```python
from build123d import *

# Parameters (mm, degrees)
SKETCH1_W            = 100
SKETCH1_H            = 100
BOSS_EXTRUDE1_DEPTH  = 5
SKETCH2_W            = 90
SKETCH2_H            = 90
SKETCH2_W_2          = 84
SKETCH2_H_2          = 84
BOSS_EXTRUDE2_DEPTH  = 10
SKETCH4_W            = 5
SKETCH4_H            = 5
SKETCH4_R            = 1.5
BOSS_EXTRUDE3_DEPTH  = 2
FILLET1_R            = 1
SKETCH5_W            = 60
SKETCH5_H            = 10
CUT_EXTRUDE1_DEPTH   = 5
SKETCH6_R            = 1.5
CUT_EXTRUDE2_DEPTH   = 5
LPATTERN1_COUNT      = 2
LPATTERN1_PITCH      = 95
LPATTERN1_COUNT_DIR2 = 2
LPATTERN1_PITCH_DIR2 = 95


with BuildPart() as part:
    # Sketch1 → Boss-Extrude1 (new body)
    with BuildSketch(Plane(origin=(0, 0, 0), x_dir=(1, 0, 0), z_dir=(0, 1, 0))):
        with Locations((50, 50)):
            Rectangle(SKETCH1_W, SKETCH1_H)
    extrude(amount=BOSS_EXTRUDE1_DEPTH)

    # Sketch2 → Boss-Extrude2 (add)
    with BuildSketch(Plane(origin=(0, 5, 0), x_dir=(1, 0, 0), z_dir=(0, 1, 0))):
        with Locations((50, 50)):
            Rectangle(SKETCH2_W, SKETCH2_H)
        with Locations((50, 50)):
            Rectangle(SKETCH2_W_2, SKETCH2_H_2, mode=Mode.SUBTRACT)
    extrude(amount=BOSS_EXTRUDE2_DEPTH)

    # Sketch4 → Boss-Extrude3 (add)
    with BuildSketch(Plane(origin=(0, 5, 0), x_dir=(1, 0, 0), z_dir=(0, 1, 0))):
        with Locations((20.54, 46.44)):
            Rectangle(SKETCH4_W, SKETCH4_H)
        with Locations((20.54, 46.44)):
            Circle(SKETCH4_R, mode=Mode.SUBTRACT)
        with Locations((20.54, 74.38)):
            Rectangle(SKETCH4_W, SKETCH4_H)
        with Locations((20.54, 74.38)):
            Circle(SKETCH4_R, mode=Mode.SUBTRACT)
        with Locations((72.61, 79.46)):
            Rectangle(SKETCH4_W, SKETCH4_H)
        with Locations((72.61, 79.46)):
            Circle(SKETCH4_R, mode=Mode.SUBTRACT)
        with Locations((71.34, 31.2)):
            Rectangle(SKETCH4_W, SKETCH4_H)
        with Locations((71.34, 31.2)):
            Circle(SKETCH4_R, mode=Mode.SUBTRACT)
    extrude(amount=BOSS_EXTRUDE3_DEPTH)

    # Fillet1
    fillet1_edges = [part.edges().sort_by_distance(p)[0] for p in [
        (8, 5, -50),
        (50, 5, -8),
        (92, 5, -50),
        (50, 5, -92),
        (23.04, 5, -74.38),
        (20.54, 5, -76.88),
        (18.04, 5, -74.38),
        (20.54, 5, -71.88),
        (75.11, 5, -79.46),
        (72.61, 5, -81.96),
        (70.11, 5, -79.46),
        (72.61, 5, -76.96),
        (23.04, 5, -46.44),
        (20.54, 5, -48.94),
        (18.04, 5, -46.44),
        (20.54, 5, -43.94),
        (73.84, 5, -31.2),
        (71.34, 5, -33.7),
        (68.84, 5, -31.2),
        (71.34, 5, -28.7),
    ]]
    fillet(fillet1_edges, radius=FILLET1_R)

    # Sketch5 → Cut-Extrude1 (cut)
    with BuildSketch(Plane(origin=(95, 0, 0), x_dir=(0, 0, -1), z_dir=(1, 0, 0))):
        with Locations((55, 10)):
            Rectangle(SKETCH5_W, SKETCH5_H)
    extrude(amount=-CUT_EXTRUDE1_DEPTH, mode=Mode.SUBTRACT)

    # Sketch6 → Cut-Extrude2 (cut)
    with BuildSketch(Plane.XZ):
        with Locations((2.5, -2.5)):
            Circle(SKETCH6_R)
    cut_extrude2 = extrude(amount=-CUT_EXTRUDE2_DEPTH, mode=Mode.SUBTRACT)

    # LPattern1: Cut-Extrude2 2 × 2
    with Locations(*[(i * LPATTERN1_PITCH, 0, -j * LPATTERN1_PITCH_DIR2) for i in range(LPATTERN1_COUNT) for j in range(LPATTERN1_COUNT_DIR2) if (i, j) != (0, 0)]):
        add(cut_extrude2, mode=Mode.SUBTRACT)


solid = part.part
```
Can you work these out from the model? Positions are in its coordinate system, mm. A direction names the side the tool comes from. Give positions to 0.01 mm unless a question says otherwise; leave off trailing zeros. Order: outer loops, then holes, each group sorted by start corner. A loop starts at its lowest first (then second) coordinate and runs counter-clockwise, first axis right, second up. Notation, with made-up numbers: M 71,-23 L 104,-23 A34 cw 104,12 Z; hole C -30,19 d2. An arc over 180 degrees is marked long. One line per item, written item: value.
1) For P1, Ø1.1, axis at y = 6.5, z = -75.5, coming from the -X side; P2, Ø3, axis at x = 75, y = 9.5, coming from the -Z side; P3, Ø1.5, axis at x = 72.5, z = -79.5, coming from the +Y side; P4, Ø2.5, axis at x = 97.5, z = -2.5, coming from the +Y side, each with a flat end and sliding along its axis, tell me the tip position at first contact or that it passes through.
Answer sheet:
P1: stops at x = 5
P2: stops at z = -95
P3: stops at y = 5
P4: passes through
2) Please list where these lines run through material, in increasing order: line 1 along X through (y, z) = (1.35, -97.5); line 2 along Z through (x, y) = (20.54, 6.55); line 3 along Z through (x, y) = (97.5, 2.8).
Answer sheet:
line 1: x = 0 to 1, 4 to 96, 99 to 100
line 2: z = -95 to -92, -76.88 to -75.88, -72.88 to -71.88, -48.94 to -47.94, -44.94 to -43.94, -8 to -5
line 3: z = -100 to -99, -96 to -4, -1 to 0
3) I want a section at B-B, the plane x = 97.5. List the corners of the cut face in (y, z) for me, plus the area to 3 significant figures.
Answer sheet:
outline: M 0,-100 L 5,-100 L 5,-99 L 0,-99 Z; M 0,-96 L 5,-96 L 5,-4 L 0,-4 Z; M 0,-1 L 5,-1 L 5,0 L 0,0 Z
area: 470 mm^2
4) I want a section at D-D, the plane x = 58. List the corners of the cut face in (y, z) for me.
Answer sheet:
outline: M 0,-100 L 5,-100 L 5,-95 L 15,-95 L 15,-92 L 6,-92 A1 cw 5,-91 L 5,-9 A1 cw 6,-8 L 15,-8 L 15,-5 L 5,-5 L 5,0 L 0,0 Z
5) I want a section at C-C, the plane z = -46.44. List the corners of the cut face in (x, y) for me, plus the area to 3 significant figures.
Answer sheet:
outline: M 0,0 L 100,0 L 100,5 L 24.04,5 A1 cw 23.04,6 L 23.04,7 L 22.04,7 L 22.04,5 L 19.04,5 L 19.04,7 L 18.04,7 L 18.04,6 A1 cw 17.04,5 L 9,5 A1 cw 8,6 L 8,15 L 5,15 L 5,5 L 0,5 Z
area: 535 mm^2
6) I want a section at A-A, the plane z = -97.5. List the corners of the cut face in (x, y) for me, plus the area to 3 significant figures.
Answer sheet:
outline: M 0,0 L 1,0 L 1,5 L 0,5 Z; M 4,0 L 96,0 L 96,5 L 4,5 Z; M 99,0 L 100,0 L 100,5 L 99,5 Z
area: 470 mm^2
7) We'd pull the mould along X, two halves only. Please class faces 4 (the face through (49, 10, -5)), 5 (the face through (0, 2, -49)), 6 (the face through (21.23, 5.99, -73.05)): released by +X, released by -X, zero draft, split by the parting line, or undercut.
Answer sheet:
face 4: zero draft
face 5: released by -X
face 6: undercut
8) On a 3-axis mill with a long thin cutter (end or side, diameter ignored), from which of +Z, -Z, +X, -X, +Y, -Y can I reach the whole of each face in a straight line? I mean faces 1 (the face through (19, 7, -73)), 2 (the face through (95, 10, -15)), 3 (the face through (21, 5, -46)). Say none if no direction works.
Answer sheet:
face 1: +X, +Y
face 2: +Z, -Z, +X, +Y
face 3: +Y
